Source: CAD feature listing. Evaluate the final solid. Frame: model axes, mm. Face numbers are marked on the shaded views. A direction names the side the tool comes from. Round coordinates to 2 decimals unless told otherwise and drop trailing zeros. Loops run counter-clockwise (first coordinate to the right, second up) from the corner with the lowest first, then second, coordinate; pieces in that order, holes last. Notation, with made-up numbers: M 47,-40 L 72,-40 A7 ccw 72,-30 Z; hole C 87,63.5 d2. An arc over 180 degrees is marked long. Write each question's results on one line, items separated by ' | '. Start each with the question number.
1. Ray query, line 1 (Z direction, x = -4, y = 0); line 2 (Y direction, x = -46, z = 34); line 3 (X direction, y = 30.5, z = 75). Return the intervals inside material, ascending.
2. Set-up query: the marked faces 4, 5, 6, 7 and 8. Return all of +Z, -Z, +X, -X, +Y, -Y with unobstructed straight access to the full face (end or side cutting, diameter ignored); none if empty.
3. Section C-C on z = 68. Output: boundary loops of the cut face in (x, y), and give its area (3 significant figures).
4. Contact query for flat-ended pins moving along their axis: pin 1 Ø5 at (x, y) = (-44, -47.5) entering from -Z; pin 2 Ø16 at (y, z) = (-5, 107) entering from -X; pin 3 Ø5 at (x, z) = (-71, 29) entering from -Y; pin 4 Ø3 at (x, z) = (-71.5, 29.5) entering from +Y. Output: stop coordinate, or through.
5. Section A-A on y = 0. Output: boundary loops of the cut face in (x, z) (3 decimals).
6. Draft query along Y for the marked faces 1, 2 and 3. Return one class per face: released by +Y, released by -Y, zero draft, split by the parting line, or undercut.
7. Section D-D on x = -8. Output: boundary loops of the cut face in (y, z), and give its area (3 significant figures).
8. Section B-B on x = -35. Output: boundary loops of the cut face in (y, z).
from build123d import *

# Parameters (mm, degrees)
F1_DEPTH  = 76.2
F2_R      = 12.7
F3_DEPTH  = 76.201
F5_DEPTH  = 152.401
F6_R      = 15.875
F7_DEPTH  = 6.35
F8_R      = 38.1
F12_DEPTH = 12.7
F14_SIZE  = 1.524
F15_W     = 6.35
F15_H     = 6.35


with BuildPart() as f1:
    # F0 (on Front) → F1 (new body, symmetric)
    with BuildSketch(Plane.XZ):
        Polygon((0, 0), (0, 152.4), (-25.4, 152.4), (-25.4, 25.4), (-76.2, 25.4), (-76.2, 0), align=None)
    extrude(amount=F1_DEPTH, both=True)

    # F2 (on face) → F3 (cut, through all)
    with BuildSketch(Plane.YZ):
        with Locations((0, 114.3)):
            Circle(F2_R)
    extrude(amount=-F3_DEPTH, mode=Mode.SUBTRACT)

    # F4 (on face) → F5 (cut, through all)
    with BuildSketch(Plane(origin=(0, 0, 0), x_dir=(1, 0, 0), z_dir=(0, 0, -1))):
        with BuildLine():
            Line((-63.5, 12.7), (-76.2, 12.7))
            Line((-76.2, 12.7), (-76.2, -12.7))
            Line((-76.2, -12.7), (-63.5, -12.7))
            ThreePointArc((-63.5, -12.7), (-50.8, 0), (-63.5, 12.7))
        make_face()
    extrude(amount=-F5_DEPTH, mode=Mode.SUBTRACT)

    # F6 (on face) → F7 (cut)
    with BuildSketch(Plane(origin=(-25.4, 0, 0), x_dir=(0, -1, 0), z_dir=(-1, 0, 0))):
        with Locations((0, 114.3)):
            Circle(F6_R)
    extrude(amount=-F7_DEPTH, mode=Mode.SUBTRACT)

    # F8
    f8_edges = [f1.edges().sort_by_distance(p)[0] for p in [
        (-12.7, -76.2, 152.4),
        (-12.7, 76.2, 152.4),
    ]]
    fillet(f8_edges, radius=F8_R)

    # F11 (on offset) → F12 (join)
    with BuildSketch(Plane.XZ.offset(44.45)):
        Polygon((-25.4, 25.4), (-25.4, 101.6), (-50.8, 25.4), align=None)
    extrude(amount=F12_DEPTH)

    # F13: F1 across plane


with BuildPart() as f1_1:
    add(f1.part)
    add(f1.part.mirror(Plane.XZ))

    # F14
    f14_edges = [f1_1.edges().sort_by_distance(p)[0] for p in [
        (-25.4, 15.875, 114.3),
        (-19.05, -12.7, 114.3),
    ]]
    chamfer(f14_edges, length=F14_SIZE)

    # F16: sweep along a path in F16_path
    with BuildLine(Plane(origin=(-63.5, 12.7, 25.4), x_dir=(0, 1, 0), z_dir=(0, 0, 1))) as f16_path:
        Line((0, 12.7), (0, 0))
        ThreePointArc((0, 0), (-12.7, -12.7), (-25.4, 0))
        Line((-25.4, 0), (-25.4, 12.7))
    # F15 (on face) → F16 (sweep)
    with BuildSketch(Plane(origin=(-76.2, 0, 0), x_dir=(0, -1, 0), z_dir=(-1, 0, 0))):
        with Locations((-15.875, 28.575)):
            Rectangle(F15_W, F15_H)
    sweep(path=f16_path.line)


solid = f1_1.part
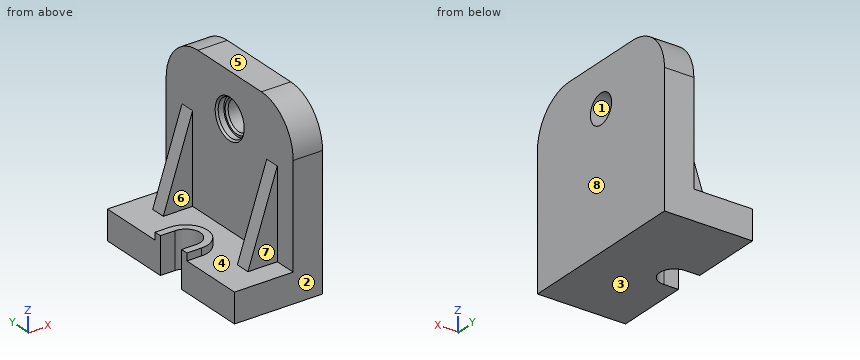
Taken from the geometry:
1) line 1: 0 to 101.6, 127 to 152.4 | line 2: -57.15 to -44.45, 44.45 to 57.15 | line 3: -25.4 to 0
2) face 4: +Z | face 5: +Z, +X, -X, +Y, -Y | face 6: +Z, -X | face 7: +Z, -X, -Y | face 8: +Z, -Z, +X, +Y, -Y
3) outline: M -36.6,-57.15 L -25.4,-57.15 L -25.4,-76.2 L 0,-76.2 L 0,76.2 L -25.4,76.2 L -25.4,57.15 L -36.6,57.15 L -36.6,44.45 L -25.4,44.45 L -25.4,-44.45 L -36.6,-44.45 Z | area: 4,160 mm^2
4) pin 1: z = 0 | pin 2: x = -24.85 | pin 3: y = -19.05 | pin 4: y = 19.05
5) outline: M -50.8,0 L 0,0 L 0,101.6 L -17.526,101.6 L -19.05,100.076 L -19.05,98.425 L -23.876,98.425 L -25.4,96.901 L -25.4,25.4 L -44.45,25.4 L -44.45,31.75 L -50.8,31.75 Z; M -25.4,131.699 L -23.876,130.175 L -19.05,130.175 L -19.05,128.524 L -17.526,127 L 0,127 L 0,152.4 L -25.4,152.4 Z
6) face 1: undercut | face 2: released by -Y | face 3: zero draft
7) outline: M -76.2,0 L 76.2,0 L 76.2,114.3 A38.1 ccw 38.1,152.4 L -38.1,152.4 A38.1 ccw -76.2,114.3 Z; hole C 0,114.3 d25.4 | area: 22,100 mm^2
8) outline: M -76.2,0 L 76.2,0 L 76.2,25.4 L 57.15,25.4 L 57.15,72.8 L 44.45,72.8 L 44.45,25.4 L -44.45,25.4 L -44.45,72.8 L -57.15,72.8 L -57.15,25.4 L -76.2,25.4 Z
